Part print with two shaded views. Sizes in mm from the minimum x, y, z corner. Coordinates: 2 decimals unless noted, no trailing zeros. Write each loop counter-clockwise with the first axis right and the second up, starting at its lowest first coordinate (ties: lowest second). Pieces come first, ordered by that corner, then holes.
Q1. Band-saw the part on D-D, the plane y = 5. Write the cut outline in (x, z), plus the area to 3 significant figures.
Q2. Band-saw the part on A-A, the plane y = 25. Write the cut outline in (x, z).
Q3. Band-saw the part on C-C, the plane x = 32.5. Write the cut outline in (y, z), plus the area to 3 significant figures.
Q4. Drill centre lines: probe 1 along Y at (x, z) = (25, 19.25); probe 2 along Z at (x, y) = (35, 7.5); probe 3 along X at (y, z) = (33, 25). Where is each one in solid material? Low to high.
Q5. Band-saw the part on B-B, the plane z = 15.25. Write the cut outline in (x, y), plus the area to 3 significant figures.
Q6. Pin check, flat tips, straight feed: P1, Ø2, axis at x = 17.5, z = 15, coming from the +Y side; P2, Ø10, axis at x = 22, z = 5.5, coming from the -Y side; P3, Ø12, axis at y = 36.5, z = 23, coming from the +X side; P4, Ø10, axis at y = 13, z = 20, coming from the +X side. Stop position of each tip, or through.
Q7. Pull direction Z, two halves, no side cores. Call the marked faces 1, 2 and 3: released by +Z, released by -Z, zero draft, split by the parting line, or undercut.
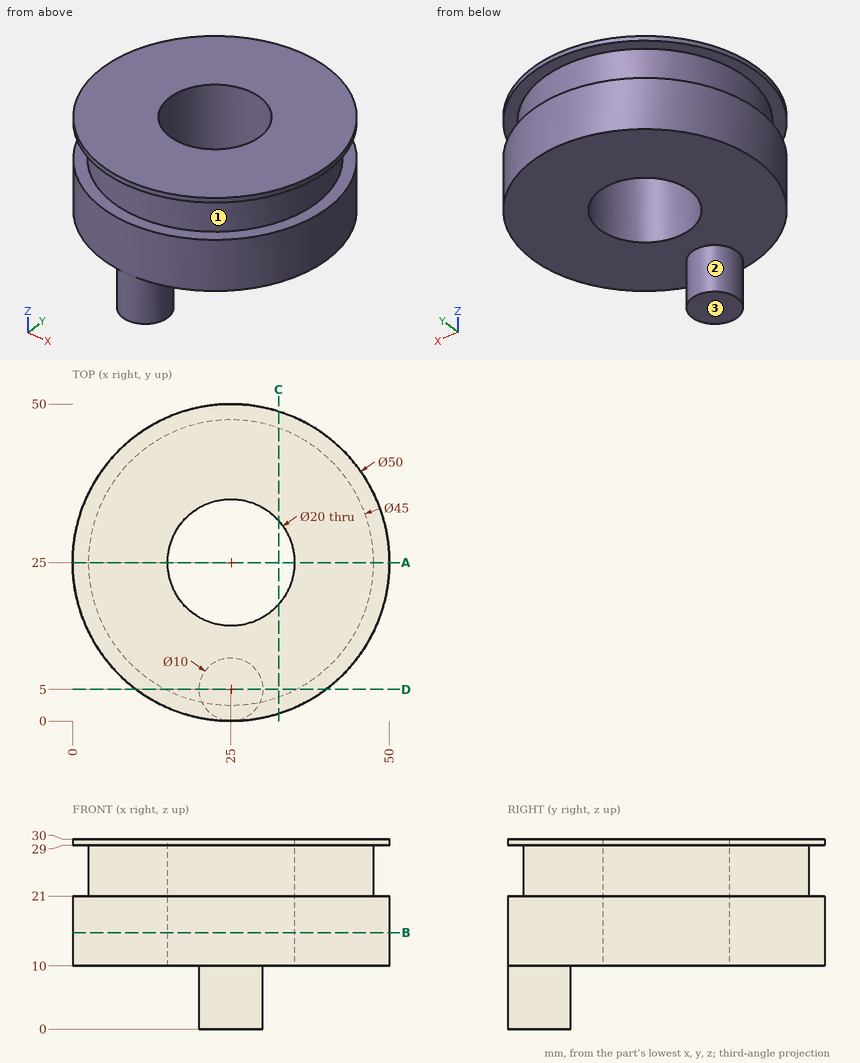
Answer sheet:
1. outline: (10, 10) - (20, 10) - (20, 0) - (30, 0) - (30, 10) - (40, 10) - (40, 21) - (35.31, 21) - (35.31, 29) - (40, 29) - (40, 30) - (10, 30) - (10, 29) - (14.69, 29) - (14.69, 21) - (10, 21) - close
1. area: 625 mm2
2. outline: (0, 10) - (15, 10) - (15, 30) - (0, 30) - (0, 29) - (2.5, 29) - (2.5, 21) - (0, 21) - close; (35, 10) - (50, 10) - (50, 21) - (47.5, 21) - (47.5, 29) - (50, 29) - (50, 30) - (35, 30) - close
3. outline: (1.15, 10) - (18.39, 10) - (18.39, 30) - (1.15, 30) - (1.15, 29) - (3.79, 29) - (3.79, 21) - (1.15, 21) - close; (31.61, 10) - (48.85, 10) - (48.85, 21) - (46.21, 21) - (46.21, 29) - (48.85, 29) - (48.85, 30) - (31.61, 30) - close
3. area: 647 mm2
4. probe 1: y = 0 to 15, 35 to 50
4. probe 2: z = 10 to 30
4. probe 3: x = 3.97 to 19, 31 to 46.03
5. outline: circle Ø50 at (25, 25); hole circle Ø20 at (25, 25)
5. area: 1,650 mm2
6. P1: stops at y = 49.14
6. P2: stops at y = 0
6. P3: stops at x = 49.31
6. P4: stops at x = 49
7. face 1: undercut
7. face 2: zero draft
7. face 3: released by -Z
